```python
from build123d import *

# Parameters (mm, degrees)
SKETCH1_R           = 50
BOSS_EXTRUDE1_DEPTH = 10
SKETCH2_R           = 50
SKETCH2_R_2         = 46.5
BOSS_EXTRUDE2_DEPTH = 1
SKETCH3_R           = 47
CUT_EXTRUDE1_DEPTH  = 7
SKETCH4_R           = 3.15
BOSS_EXTRUDE3_DEPTH = 7


with BuildPart() as part:
    # Sketch1 → Boss-Extrude1 (new body)
    with BuildSketch(Plane(origin=(0, 0, 0), x_dir=(1, 0, 0), z_dir=(0, 1, 0))):
        Circle(SKETCH1_R)
    extrude(amount=BOSS_EXTRUDE1_DEPTH)

    # Sketch2 → Boss-Extrude2 (add)
    with BuildSketch(Plane(origin=(0, 10, 0), x_dir=(1, 0, 0), z_dir=(0, 1, 0))):
        Circle(SKETCH2_R)
        Circle(SKETCH2_R_2, mode=Mode.SUBTRACT)
    extrude(amount=BOSS_EXTRUDE2_DEPTH)

    # Sketch3 → Cut-Extrude1 (cut)
    with BuildSketch(Plane.XZ):
        Circle(SKETCH3_R)
    extrude(amount=-CUT_EXTRUDE1_DEPTH, mode=Mode.SUBTRACT)

    # Sketch4 → Boss-Extrude3 (add)
    with BuildSketch(Plane(origin=(0, 0, 0), x_dir=(1, 0, 0), z_dir=(0, 1, 0))):
        with BuildLine():
            Line((-47.696960071, 15), (-70, 15))
            Line((-70, 15), (-70, -15))
            Line((-70, -15), (-47.696960071, -15))
            ThreePointArc((-47.696960071, -15), (-50, 0), (-47.696960071, 15))
        make_face()
        with Locations((-60, 0)):
            Circle(SKETCH4_R, mode=Mode.SUBTRACT)
        with BuildLine():
            Line((47.696960071, -15), (70, -15))
            Line((70, -15), (70, 15))
            Line((70, 15), (47.696960071, 15))
            ThreePointArc((47.696960071, 15), (50, 0), (47.696960071, -15))
        make_face()
        with Locations((60, 0)):
            Circle(SKETCH4_R, mode=Mode.SUBTRACT)
    extrude(amount=BOSS_EXTRUDE3_DEPTH)


solid = part.part
```
The model under review builds one solid part; all positions refer to its coordinate system, in mm. A direction names the side the tool comes from. Coordinates: 2 decimals unless noted, no trailing zeros. Order: outer loops, then holes, each group sorted by start corner. A loop starts at its lowest first (then second) coordinate and runs counter-clockwise, first axis right, second up. Notation, with made-up numbers: (-24, 89) -> (-14, 89) arc R34 cw to (-14, 126) -> close; hole circle Ø9 at (4.25, -37.75). An arc over 180 degrees is marked (long way). Answer in a Markdown table with one row per item. Add a question column.
Item 1: To check wall thickness, follow probe 1 along Z at (x, y) = (0, 1.75); probe 2 along Z at (x, y) = (-60, 4.5); probe 3 along Y at (x, z) = (31.5, -23.5). State the ranges of each line that lie inside material, in increasing order.
Item 2: We need section C-C on y = 3.5. Write out the cut boundary in (x, z), plus the area to 3 significant figures.
Item 3: We need section D-D on x = 0. Write out the cut boundary in (y, z).
Item 4: We need section A-A on x = 60. Write out the cut boundary in (y, z), plus the area to 3 significant figures.
Item 5: We need section B-B on z = 0. Write out the cut boundary in (x, y).
Item 6: Mouldability with a two-part tool opening along Z and no side actions: class faces 1 (the flat face through (59, 3, -15)), 2 (the flat face through (-59, 3, 15)), 3 (the cylindrical face through (-63.147, 3.451, -0.138)), 4 (the flat face through (56, 7, 0)) as +Z half, -Z half, draft (parallel to the pull), parting line (faces both ways), or undercut.
Item 7: Clearance check with flat-ended pins moving along their axes: pin 1 (1.5 mm diameter, centred on y = 1.5, z = -38.5, fed in from +X); pin 2 (1 mm diameter, centred on x = 46, y = 4, fed in from -Z); pin 3 (11 mm diameter, centred on x = -58.5, z = 2.5, fed in from +Y); pin 4 (5 mm diameter, centred on x = 60, z = 0, fed in from -Y). State where each tip first meets the part, or that it passes through.
Item 8: Machinability: for faces 5 (the flat face through (-59, 3, -15)), 6 (the flat face through (-1, 10, -1)), 7 (the flat face through (59, 3, 15)), 8 (the cylindrical face through (44.83, 3.45, 14.12)), which of the approach directions +Z, -Z, +X, -X, +Y, -Y give a long, thin tool a straight path to every point of the face, cutting with its end or side? Answer none if there is none.
Final values:
| question | item | result |
|---|---|---|
| 1 | probe 1 | z = -50 to -47, 47 to 50 |
| 1 | probe 2 | z = -15 to -3.15, 3.15 to 15 |
| 1 | probe 3 | y = 7 to 10 |
| 2 | outline | (-70, -15) -> (-47.7, -15) arc R50 ccw to (47.7, -15) -> (70, -15) -> (70, 15) -> (47.7, 15) arc R50 ccw to (-47.7, 15) -> (-70, 15) -> close; hole circle Ø6.3 at (-60, 0); hole circle Ø94 at (0, 0); hole circle Ø6.3 at (60, 0) |
| 2 | area | 2,100 mm2 |
| 3 | outline | (0, -50) -> (11, -50) -> (11, -46.5) -> (10, -46.5) -> (10, 46.5) -> (11, 46.5) -> (11, 50) -> (0, 50) -> (0, 47) -> (7, 47) -> (7, -47) -> (0, -47) -> close |
| 4 | outline | (0, -15) -> (7, -15) -> (7, -3.15) -> (0, -3.15) -> close; (0, 3.15) -> (7, 3.15) -> (7, 15) -> (0, 15) -> close |
| 4 | area | 166 mm2 |
| 5 | outline | (-70, 0) -> (-63.15, 0) -> (-63.15, 7) -> (-70, 7) -> close; (-56.85, 0) -> (-47, 0) -> (-47, 7) -> (47, 7) -> (47, 0) -> (56.85, 0) -> (56.85, 7) -> (50, 7) -> (50, 11) -> (46.5, 11) -> (46.5, 10) -> (-46.5, 10) -> (-46.5, 11) -> (-50, 11) -> (-50, 7) -> (-56.85, 7) -> close; (63.15, 0) -> (70, 0) -> (70, 7) -> (63.15, 7) -> close |
| 6 | face 1 | -Z half |
| 6 | face 2 | +Z half |
| 6 | face 3 | undercut |
| 6 | face 4 | draft |
| 7 | pin 1 | stops at x = 32.79 |
| 7 | pin 2 | stops at z = -20.73 |
| 7 | pin 3 | stops at y = 7 |
| 7 | pin 4 | passes through |
| 8 | face 5 | -Z, -X, +Y, -Y |
| 8 | face 6 | +Y |
| 8 | face 7 | +Z, +X, +Y, -Y |
| 8 | face 8 | -Y |
